```python
from build123d import *

# Parameters (mm, degrees)
BOSS_EXTRUDE1_DEPTH = 5


with BuildPart() as part:
    # Sketch1 → Boss-Extrude1 (new body)
    with BuildSketch(Plane(origin=(0, 0, 0), x_dir=(0, 0, -1), z_dir=(1, 0, 0))):
        with BuildLine():
            Line((2.5, 29.895651858), (2.5, 24.874685928))
            ThreePointArc((2.5, 24.874685928), (18.540496218, 16.770509831), (25, 0))
            ThreePointArc((25, 0), (24.441795639, -5.253439439), (22.792109925, -10.272279454))
            Line((22.792109925, -10.272279454), (27.140393972, -12.782762419))
            ThreePointArc((27.140393972, -12.782762419), (29.276371182, -6.549358016), (30, 0))
            ThreePointArc((30, 0), (22.079402166, 20.310096012), (2.5, 29.895651858))
        make_face()
        with BuildLine():
            ThreePointArc((-22.792109925, -10.272279454), (-21.650635095, 12.5), (-2.5, 24.874685928))
            Line((-2.5, 24.874685928), (-2.5, 29.895651858))
            ThreePointArc((-2.5, 29.895651858), (-25.980762114, 15), (-27.140393972, -12.782762419))
            Line((-27.140393972, -12.782762419), (-22.792109925, -10.272279454))
        make_face()
        with BuildLine():
            Line((-2.5, 29.895651858), (-2.5, 24.874685928))
            ThreePointArc((-2.5, 24.874685928), (0, 25), (2.5, 24.874685928))
            Line((2.5, 24.874685928), (2.5, 29.895651858))
            ThreePointArc((2.5, 29.895651858), (0, 30), (-2.5, 29.895651858))
        make_face()
        with BuildLine():
            ThreePointArc((22.792109925, -10.272279454), (21.650635095, -12.5), (20.292109925, -14.602406473))
            Line((20.292109925, -14.602406473), (24.640393972, -17.112889438))
            ThreePointArc((24.640393972, -17.112889438), (25.980762114, -15), (27.140393972, -12.782762419))
            Line((27.140393972, -12.782762419), (22.792109925, -10.272279454))
        make_face()
        with BuildLine():
            ThreePointArc((20.292109925, -14.602406473), (0, -25), (-20.292109925, -14.602406473))
            Line((-20.292109925, -14.602406473), (-24.640393972, -17.112889438))
            ThreePointArc((-24.640393972, -17.112889438), (0, -30), (24.640393972, -17.112889438))
            Line((24.640393972, -17.112889438), (20.292109925, -14.602406473))
        make_face()
        with BuildLine():
            ThreePointArc((-20.292109925, -14.602406473), (-21.650635095, -12.5), (-22.792109925, -10.272279454))
            Line((-22.792109925, -10.272279454), (-27.140393972, -12.782762419))
            ThreePointArc((-27.140393972, -12.782762419), (-25.980762114, -15), (-24.640393972, -17.112889438))
            Line((-24.640393972, -17.112889438), (-20.292109925, -14.602406473))
        make_face()
        with BuildLine():
            Line((7.5, -4.330127019), (5, -5.773502692))
            Line((5, -5.773502692), (20.292109925, -14.602406473))
            ThreePointArc((20.292109925, -14.602406473), (21.650635095, -12.5), (22.792109925, -10.272279454))
            Line((22.792109925, -10.272279454), (7.5, -1.443375673))
            Line((7.5, -1.443375673), (7.5, -4.330127019))
        make_face()
        with BuildLine():
            Line((-7.5, -4.330127019), (-7.5, -1.443375673))
            Line((-7.5, -1.443375673), (-22.792109925, -10.272279454))
            ThreePointArc((-22.792109925, -10.272279454), (-21.650635095, -12.5), (-20.292109925, -14.602406473))
            Line((-20.292109925, -14.602406473), (-5, -5.773502692))
            Line((-5, -5.773502692), (-7.5, -4.330127019))
        make_face()
        with BuildLine():
            Line((-2.5, 24.874685928), (-2.5, 7.216878365))
            Line((-2.5, 7.216878365), (0, 8.660254038))
            Line((0, 8.660254038), (2.5, 7.216878365))
            Line((2.5, 7.216878365), (2.5, 24.874685928))
            ThreePointArc((2.5, 24.874685928), (0, 25), (-2.5, 24.874685928))
        make_face()
        Polygon((-5, 2.886751346), (-2.5, 4.330127019), (-2.5, 7.216878365), (-7.5, 4.330127019), (-7.5, -1.443375673), (-5, 0), align=None)
        Polygon((-2.5, 7.216878365), (-2.5, 4.330127019), (0, 5.773502692), (2.5, 4.330127019), (2.5, 7.216878365), (0, 8.660254038), align=None)
        Polygon((2.5, 7.216878365), (2.5, 4.330127019), (5, 2.886751346), (5, 0), (7.5, -1.443375673), (7.5, 4.330127019), align=None)
        Polygon((5, -2.886751346), (2.5, -4.330127019), (5, -5.773502692), (7.5, -4.330127019), (7.5, -1.443375673), (5, 0), align=None)
        Polygon((5, -5.773502692), (2.5, -4.330127019), (0, -5.773502692), (-2.5, -4.330127019), (-5, -5.773502692), (0, -8.660254038), align=None)
        Polygon((-5, -2.886751346), (-5, 0), (-7.5, -1.443375673), (-7.5, -4.330127019), (-5, -5.773502692), (-2.5, -4.330127019), align=None)
    extrude(amount=BOSS_EXTRUDE1_DEPTH)


solid = part.part
```
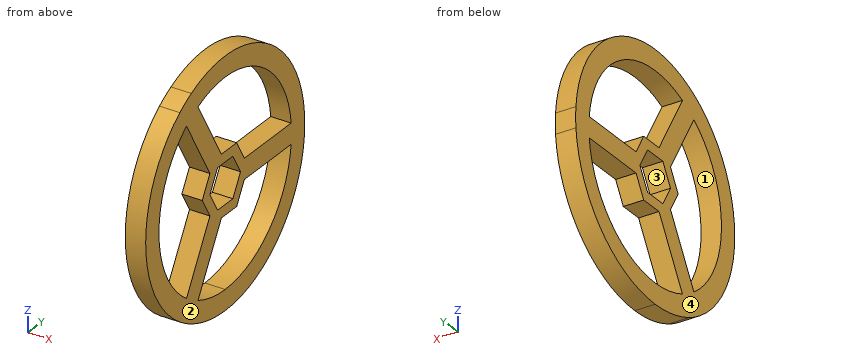
Work out the finished part from the listing and answer in its coordinate system (mm). Face numbers are marked on the shaded views. A direction names the side the tool comes from. Coordinates: 2 decimals unless noted, no trailing zeros. Order: outer loops, then holes, each group sorted by start corner. A loop starts at its lowest first (then second) coordinate and runs counter-clockwise, first axis right, second up. Notation, with made-up numbers: (-20.5, -34) - (0.5, -34) arc R12 cw to (0.5, -29) - close; hole circle Ø1 at (46, 37). An arc over 180 degrees is marked (long way). Answer as a JSON object with one key per item and string values.
1. A tool of negligible diameter and unlimited length cuts with its end or side. For the marked faces 1 and 2, from which of +Z, -Z, +X, -X, +Y, -Y can it reach the whole face along a straight path? Write none if from no direction.
Output values:
{"face 1": "+X, -X", "face 2": "+Z, -Z, +X, +Y, -Y"}
2. Find section A-A on x = 1.6. Determine the outline of the cut face in (y, z), plus the area to 3 significant figures.
Output values:
{"outline": "circle Ø60 at (0, 0); hole (-14.6, -20.29) - (-5.77, -5) - (-8.66, 0) - (-5.77, 5) - (-14.6, 20.29) arc R25 ccw to start; hole (-10.27, -22.79) arc R25 ccw to (24.87, -2.5) - (7.22, -2.5) - (4.33, -7.5) - (-1.44, -7.5) - close; hole (-10.27, 22.79) - (-1.44, 7.5) - (4.33, 7.5) - (7.22, 2.5) - (24.87, 2.5) arc R25 ccw to start; hole (-5.77, 0) - (-2.89, -5) - (2.89, -5) - (5.77, 0) - (2.89, 5) - (-2.89, 5) - close", "area": "1,230 mm²"}
3. Find section B-B on z = 23.5. Determine the outline of the cut face in (x, y), plus the area to 3 significant figures.
Output values:
{"outline": "(0, -18.65) - (5, -18.65) - (5, -8.53) - (0, -8.53) - close; (0, 8.53) - (5, 8.53) - (5, 18.65) - (0, 18.65) - close", "area": "101 mm²"}
4. Find section C-C on y = -18. Determine the outline of the cut face in (x, z).
Output values:
{"outline": "(0, -24) - (5, -24) - (5, -17.35) - (0, -17.35) - close; (0, 17.35) - (5, 17.35) - (5, 24) - (0, 24) - close"}
5. Find section D-D on y = 11.5. Determine the outline of the cut face in (x, z).
Output values:
{"outline": "(0, -27.71) - (5, -27.71) - (5, -22.2) - (0, -22.2) - close; (0, -2.5) - (5, -2.5) - (5, 2.5) - (0, 2.5) - close; (0, 22.2) - (5, 22.2) - (5, 27.71) - (0, 27.71) - close"}
6. The mould has two halves that part along Y. Classify the marked faces 3 and 4: +Y half, -Y half, draft (parallel to the pull), parting line (faces both ways), or undercut.
Output values:
{"face 3": "undercut", "face 4": "draft"}
7. Each of these flat-tipped pins is pushed along its axis until it touches: P1, Ø3, axis at x = 0.5, y = 20.5, coming from the +Z side; P2, Ø2.5, axis at x = 2.5, y = 17, coming from the +Z side; P3, Ø8, axis at y = -6, z = 15, coming from the -X side; P4, Ø10, axis at y = 7, z = -16.5, coming from the -X side. Where does it stop, or does it pass through?
Output values:
{"P1": "stops at z = 23.22", "P2": "stops at z = 25.53", "P3": "stops at x = 0", "P4": "passes through"}
8. Consider line 1 (Y direction, x = 3, z = 6.5); line 2 (Z direction, x = 0.95, y = 21); line 3 (Y direction, x = 2.45, z = 19). Determine where each line is inside the solid, lowest interval first.
Output values:
{"line 1": "y = -29.29 to -24.14, -6.64 to 4.91, 24.14 to 29.29", "line 2": "z = -21.42 to -13.56, -2.5 to 2.5, 13.56 to 21.42", "line 3": "y = -23.22 to -16.25, -13.86 to -8.08, 16.25 to 23.22"}
